Can you work these out from the model? Positions are in its coordinate system, mm. A direction names the side the tool comes from. Coordinates: 2 decimals unless noted, no trailing zeros. Order: outer loops, then holes, each group sorted by start corner. A loop starts at its lowest first (then second) coordinate and runs counter-clockwise, first axis right, second up. Notation, with made-up numbers: (-2.5, -24) -> (51.5, -24) arc R17 ccw to (51.5, -5) -> close; hole circle Ø10 at (21.5, 79.5). An arc over 180 degrees is marked (long way). Write item = value, one per line.
```python
from build123d import *

# Parameters (mm, degrees)
BOSS_EXTRUDE1_DEPTH = 31.75
BOSS_EXTRUDE3_DEPTH = 63.5
CUT_EXTRUDE1_DEPTH  = 175.52526199
SKETCH4_R           = 7.5
CUT_EXTRUDE2_DEPTH  = 82.140420864


with BuildPart() as part:
    # Sketch1 → Boss-Extrude1 (new, symmetric)
    with BuildSketch(Plane.XY):
        Polygon((15, 152.926386675), (-35, 152.926386675), (-35, 100.426386675), (15, 100.426386675), (15, 97.926386675), (-37.5, 97.926386675), (-37.5, 155.426386675), (15, 155.426386675), align=None)
    extrude(amount=BOSS_EXTRUDE1_DEPTH, both=True)

    # Sketch2 → Boss-Extrude3 (add)
    with BuildSketch(Plane.XY.offset(31.75)):
        Polygon((-37.5, 97.926386675), (-47.638801391, 155.426386675), (-37.5, 155.426386675), align=None)
    extrude(amount=-BOSS_EXTRUDE3_DEPTH)

    # Sketch3 → Cut-Extrude1 (cut, through all)
    with BuildSketch(Plane.XY.offset(31.75)):
        Polygon((-35, 152.926386675), (-44.257166487, 152.926386675), (-35, 100.426386675), align=None)
    extrude(amount=-CUT_EXTRUDE1_DEPTH, mode=Mode.SUBTRACT)

    # Sketch4 → Cut-Extrude2 (cut, through all)
    with BuildSketch(Plane(origin=(0, 155.426386675, 0), x_dir=(1, 0, 0), z_dir=(0, 1, 0))):
        with Locations(Location((0, 0, 0), (0, 0, 270))):
            Circle(SKETCH4_R)
    extrude(amount=-CUT_EXTRUDE2_DEPTH, mode=Mode.SUBTRACT)


solid = part.part
```
Item 1: If I drill on probe 1 along Y at (x, z) = (-17.5, -15.5); probe 2 along X at (y, z) = (153.5, 0); probe 3 along X at (y, z) = (154.2, 0), over which ranges is the centre line in solid material (lowest first)?
A:
probe_1 = 97.93 to 100.43, 152.93 to 155.43
probe_2 = -47.3 to -7.5, 7.5 to 15
probe_3 = -47.42 to -7.5, 7.5 to 15
Item 2: I want a section at D-D, the plane z = -18. Please give me the cut outline in (x, y).
A:
outline = (-47.64, 155.43) -> (-37.5, 97.93) -> (15, 97.93) -> (15, 100.43) -> (-35, 100.43) -> (-44.26, 152.93) -> (15, 152.93) -> (15, 155.43) -> close
Item 3: I want a section at A-A, the plane x = -11. Please give me the cut outline in (y, z).
A:
outline = (97.93, -31.75) -> (100.43, -31.75) -> (100.43, 31.75) -> (97.93, 31.75) -> close; (152.93, -31.75) -> (155.43, -31.75) -> (155.43, 31.75) -> (152.93, 31.75) -> close
Item 4: I want a section at B-B, the plane z = 0. Please give me the cut outline in (x, y).
A:
outline = (-47.64, 155.43) -> (-37.5, 97.93) -> (-7.5, 97.93) -> (-7.5, 100.43) -> (-35, 100.43) -> (-44.26, 152.93) -> (-7.5, 152.93) -> (-7.5, 155.43) -> close; (7.5, 97.93) -> (15, 97.93) -> (15, 100.43) -> (7.5, 100.43) -> close; (7.5, 152.93) -> (15, 152.93) -> (15, 155.43) -> (7.5, 155.43) -> close
Item 5: For faces 5 (the flat face through (-17, 155.426, 0)), 6 (the flat face through (-14, 152.926, 0)), which set-ups out of +Z, -Z, +X, -X, +Y, -Y let a thin tool reach every point of the face, with its end or its side?
A:
face_5 = +Z, -Z, +X, -X, +Y
face_6 = +Z, -Z, +X
Item 6: I'm going to push flat-ended pins straight in: P1, Ø24, axis at x = 0, z = 0, coming from the -Y side; P2, Ø4, axis at y = 117, z = -8, coming from the -X side; P3, Ø2, axis at y = 107, z = -21.5, coming from the -X side; P4, Ø5, axis at y = 124, z = 19.5, coming from the -X side. Where does each tip first touch, or does it pass through?
A:
P1 = 97.93
P2 = -41.22
P3 = -39.28
P4 = -42.54
Item 7: If we mould it in two halves opening along X, with no side actions, what happens to faces 1 (the flat face through (-10, 100.426, 0)), 2 (the cylindrical face through (0.33, 99.194, -7.493)), 3 (the flat face through (15, 99, 0)), 4 (the cylindrical face through (0.33, 154.194, -7.493))? For each: pulls with the +X half, pulls with the -X half, needs draft (parallel to the pull), parting line crosses it, or undercut.
A:
face_1 = needs draft
face_2 = undercut
face_3 = pulls with the +X half
face_4 = undercut
Item 8: I want a section at C-C, the plane x = 0. Please give me the cut outline in (y, z).
A:
outline = (97.93, -31.75) -> (100.43, -31.75) -> (100.43, -7.5) -> (97.93, -7.5) -> close; (97.93, 7.5) -> (100.43, 7.5) -> (100.43, 31.75) -> (97.93, 31.75) -> close; (152.93, -31.75) -> (155.43, -31.75) -> (155.43, -7.5) -> (152.93, -7.5) -> close; (152.93, 7.5) -> (155.43, 7.5) -> (155.43, 31.75) -> (152.93, 31.75) -> close
